Design review of the part built by this model. Coordinates are the model's own, in mm. Face numbers are marked on the shaded views. Give positions to 0.01 mm unless a question says otherwise; leave off trailing zeros. Order: outer loops, then holes, each group sorted by start corner. A loop starts at its lowest first (then second) coordinate and runs counter-clockwise, first axis right, second up.
```python
from build123d import *

# Parameters (mm, degrees)
SKETCH1_R           = 2
SKETCH1_R_2         = 50
BOSS_EXTRUDE1_DEPTH = 10
SKETCH2_R           = 21.25
CUT_EXTRUDE1_DEPTH  = 5
SKETCH2_3_R         = 1.75
CUT_EXTRUDE2_DEPTH  = 85.067442245
SKETCH4_R           = 10
CUT_EXTRUDE3_DEPTH  = 84.620182047


with BuildPart() as part:
    # Sketch1 → Boss-Extrude1 (new body)
    # profile 1 of 5: a face of its own
    with BuildSketch(Plane(origin=(0, 0, 0), x_dir=(1, 0, 0), z_dir=(0, 1, 0))):
        with BuildLine():
            ThreePointArc((-38.537319575, -55.507882323), (-26.466358431, -48.502831547), (-12.510350744, -48.409618097))
            ThreePointArc((-12.510350744, -48.409618097), (-35.355339059, -35.355339059), (-48.409618097, -12.510350744))
            ThreePointArc((-48.409618097, -12.510350744), (-48.502831547, -26.466358431), (-55.507882323, -38.537319575))
            ThreePointArc((-55.507882323, -38.537319575), (-55.507882323, -55.507882323), (-38.537319575, -55.507882323))
        make_face()
        with Locations(Location((-47.022600949, -47.022600949, 0), (0, 0, 270))):
            Circle(SKETCH1_R, mode=Mode.SUBTRACT)
    # profile 2 of 5: a face of its own
    with BuildSketch(Plane(origin=(0, 0, 0), x_dir=(1, 0, 0), z_dir=(0, 1, 0))):
        with BuildLine():
            ThreePointArc((55.507882323, -38.537319575), (48.502831547, -26.466358431), (48.409618097, -12.510350744))
            ThreePointArc((48.409618097, -12.510350744), (35.355339059, -35.355339059), (12.510350744, -48.409618097))
            ThreePointArc((12.510350744, -48.409618097), (26.466358431, -48.502831547), (38.537319575, -55.507882323))
            ThreePointArc((38.537319575, -55.507882323), (55.507882323, -55.507882323), (55.507882323, -38.537319575))
        make_face()
        with Locations(Location((47.022600949, -47.022600949, 0), (0, 0, 270))):
            Circle(SKETCH1_R, mode=Mode.SUBTRACT)
    # profile 3 of 5: a face of its own
    with BuildSketch(Plane(origin=(0, 0, 0), x_dir=(1, 0, 0), z_dir=(0, 1, 0))):
        with BuildLine():
            ThreePointArc((12.510350744, 48.409618097), (35.355339059, 35.355339059), (48.409618097, 12.510350744))
            ThreePointArc((48.409618097, 12.510350744), (48.502831547, 26.466358431), (55.507882323, 38.537319575))
            ThreePointArc((55.507882323, 38.537319575), (55.507882323, 55.507882323), (38.537319575, 55.507882323))
            ThreePointArc((38.537319575, 55.507882323), (26.466358431, 48.502831547), (12.510350744, 48.409618097))
        make_face()
        with Locations(Location((47.022600949, 47.022600949, 0), (0, 0, 270))):
            Circle(SKETCH1_R, mode=Mode.SUBTRACT)
    # profile 4 of 5: a face of its own
    with BuildSketch(Plane(origin=(0, 0, 0), x_dir=(1, 0, 0), z_dir=(0, 1, 0))):
        with BuildLine():
            ThreePointArc((-48.409618097, 12.510350744), (-35.355339059, 35.355339059), (-12.510350744, 48.409618097))
            ThreePointArc((-12.510350744, 48.409618097), (-26.466358431, 48.502831547), (-38.537319575, 55.507882323))
            ThreePointArc((-38.537319575, 55.507882323), (-55.507882323, 55.507882323), (-55.507882323, 38.537319575))
            ThreePointArc((-55.507882323, 38.537319575), (-48.502831547, 26.466358431), (-48.409618097, 12.510350744))
        make_face()
        with Locations(Location((-47.022600949, 47.022600949, 0), (0, 0, 270))):
            Circle(SKETCH1_R, mode=Mode.SUBTRACT)
    # profile 5 of 5: a face of its own
    with BuildSketch(Plane(origin=(0, 0, 0), x_dir=(1, 0, 0), z_dir=(0, 1, 0))):
        Circle(SKETCH1_R_2)
        with BuildLine():
            ThreePointArc((-28.838834765, 32.374368671), (-32.374368671, 32.374368671), (-32.374368671, 28.838834765))
            Line((-32.374368671, 28.838834765), (-21.767766953, 18.232233047))
            ThreePointArc((-21.767766953, 18.232233047), (-18.232233047, 18.232233047), (-18.232233047, 21.767766953))
            Line((-18.232233047, 21.767766953), (-28.838834765, 32.374368671))
        make_face(mode=Mode.SUBTRACT)
        with BuildLine():
            ThreePointArc((-32.374368671, -28.838834765), (-32.374368671, -32.374368671), (-28.838834765, -32.374368671))
            Line((-28.838834765, -32.374368671), (-18.232233047, -21.767766953))
            ThreePointArc((-18.232233047, -21.767766953), (-18.232233047, -18.232233047), (-21.767766953, -18.232233047))
            Line((-21.767766953, -18.232233047), (-32.374368671, -28.838834765))
        make_face(mode=Mode.SUBTRACT)
        with BuildLine():
            ThreePointArc((28.838834765, -32.374368671), (32.374368671, -32.374368671), (32.374368671, -28.838834765))
            Line((32.374368671, -28.838834765), (21.767766953, -18.232233047))
            ThreePointArc((21.767766953, -18.232233047), (18.232233047, -18.232233047), (18.232233047, -21.767766953))
            Line((18.232233047, -21.767766953), (28.838834765, -32.374368671))
        make_face(mode=Mode.SUBTRACT)
        with BuildLine():
            ThreePointArc((32.374368671, 28.838834765), (32.374368671, 32.374368671), (28.838834765, 32.374368671))
            Line((28.838834765, 32.374368671), (18.232233047, 21.767766953))
            ThreePointArc((18.232233047, 21.767766953), (18.232233047, 18.232233047), (21.767766953, 18.232233047))
            Line((21.767766953, 18.232233047), (32.374368671, 28.838834765))
        make_face(mode=Mode.SUBTRACT)
    extrude(amount=BOSS_EXTRUDE1_DEPTH)

    # Sketch2 → Cut-Extrude1 (cut)
    with BuildSketch(Plane.XZ):
        with Locations(Location((0, 0, 0), (0, 0, 270))):
            Circle(SKETCH2_R)
    extrude(amount=-CUT_EXTRUDE1_DEPTH, mode=Mode.SUBTRACT)

    # Sketch2_3 → Cut-Extrude2 (cut, through all)
    with BuildSketch(Plane.XZ):
        with Locations(Location((-12.557368355, -7.25, 0), (0, 0, 270))):
            Circle(SKETCH2_3_R)
        with Locations(Location((12.557368355, -7.25, 0), (0, 0, 270))):
            Circle(SKETCH2_3_R)
        with Locations(Location((0, 14.5, 0), (0, 0, 270))):
            Circle(SKETCH2_3_R)
    extrude(amount=-CUT_EXTRUDE2_DEPTH, mode=Mode.SUBTRACT)

    # Sketch4 → Cut-Extrude3 (cut, through all)
    with BuildSketch(Plane(origin=(0, 5, 0), x_dir=(-1, 0, 0), z_dir=(0, -1, 0))):
        with Locations(Location((0, 0, 0), (0, 0, 90))):
            Circle(SKETCH4_R)
    extrude(amount=-CUT_EXTRUDE3_DEPTH, mode=Mode.SUBTRACT)


solid = part.part
```
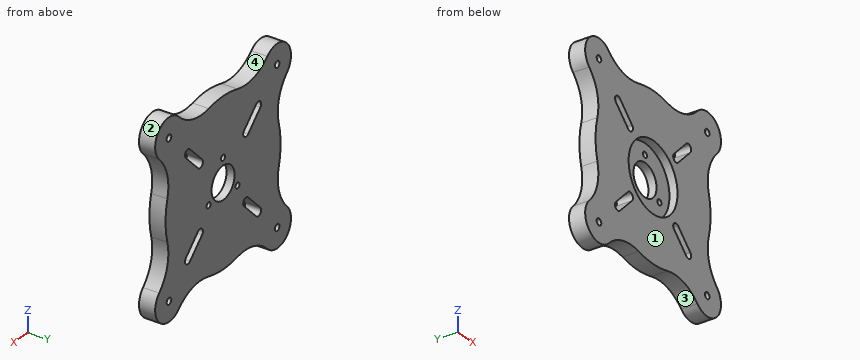
1. Take a section at A-A (z = -2.5). State the section outline as (x, y) points.
Recorded:
outline: (-49.94, 0) - (-21.1, 0) - (-21.1, 5) - (-9.68, 5) - (-9.68, 10) - (-49.94, 10) - close; (9.68, 5) - (21.1, 5) - (21.1, 0) - (49.94, 0) - (49.94, 10) - (9.68, 10) - close
2. Take a section at B-B (z = 26). State the section outline as (x, y) points.
Recorded:
outline: (-48.38, 0) - (-29.54, 0) - (-29.54, 10) - (-48.38, 10) - close; (-22.46, 0) - (22.46, 0) - (22.46, 10) - (-22.46, 10) - close; (29.54, 0) - (48.38, 0) - (48.38, 10) - (29.54, 10) - close
3. For pin 1 (1.5 mm diameter, centred on x = -32.5, y = 6, fed in from -Z); pin 2 (4 mm diameter, centred on y = 8.5, z = 4, fed in from -X); pin 3 (5 mm diameter, centred on x = -47.02, z = -47.02, fed in from +Y); pin 4 (21 mm diameter, centred on x = 8.5, z = 3.5, fed in from -Y), all flat-tipped, find the tip position at first contact; note any pin that passes through.
Recorded:
pin 1: stops at z = -51.39
pin 2: stops at x = -49.96
pin 3: stops at y = 10
pin 4: stops at y = 5
4. Draft analysis for pull direction Z (two halves, no side actions). For the marked faces 1, 2, 3 and 4, state which applies: pulls with the +Z half, pulls with the -Z half, needs draft (parallel to the pull), parting line crosses it, or undercut.
Recorded:
face 1: needs draft
face 2: undercut
face 3: pulls with the -Z half
face 4: pulls with the +Z half
5. For line 1 along X through (y, z) = (1.75, -28); line 2 along X through (y, z) = (7.6, -7.25); line 3 along Z through (x, y) = (-24.5, 7), list the stretches that pass through material, from the lowest coordinate up.
Recorded:
line 1: x = -48.97 to -31.54, -24.46 to 24.46, 31.54 to 48.97
line 2: x = -49.47 to -14.31, -10.81 to -6.89, 6.89 to 10.81, 14.31 to 49.47
line 3: z = -48.04 to -28.04, -20.96 to 20.96, 28.04 to 48.04
6. Take a section at C-C (y = 1.5). State how many separate pieces and enclosed holes the cut face has, then the cut area to 3 significant figures.
Recorded:
separate pieces: 1
enclosed holes: 9
area: 8,940 mm2
7. Take a section at D-D (x = 35). State the section outline as (y, z) points.
Recorded:
outline: (0, -52.53) - (10, -52.53) - (10, 52.53) - (0, 52.53) - close
